Geometry check sheet. Reference: the model listing, model coordinates, mm. Face numbers are marked on the shaded views. A direction names the side the tool comes from. Round coordinates to 2 decimals unless told otherwise and drop trailing zeros. Loops run counter-clockwise (first coordinate to the right, second up) from the corner with the lowest first, then second, coordinate; pieces in that order, holes last. Notation, with made-up numbers: (50.25, -23.75) - (84.25, -23.75) arc R16 cw to (84.25, -18.75) - close; hole circle Ø1 at (32.25, -33.75). An arc over 180 degrees is marked (long way). Write item = value, one per line.
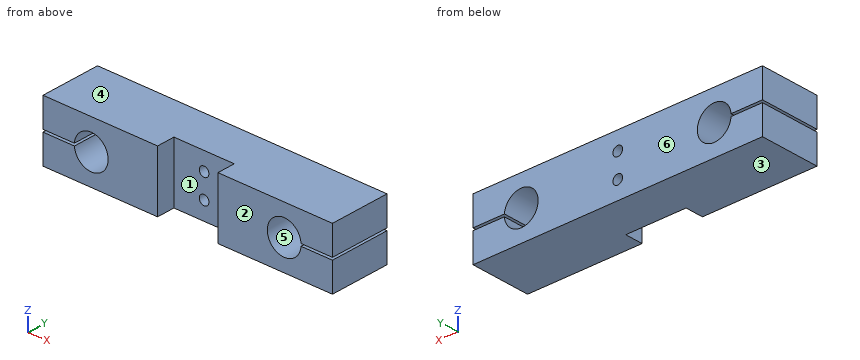
```python
from build123d import *

# Parameters (mm, degrees)
EXTRUDE_1_DEPTH     = 50
SKETCH_3_W          = 50
SKETCH_3_H          = 50
CUT_EXTRUDE_1_DEPTH = 15
SKETCH_4_R          = 4
CUT_EXTRUDE_2_DEPTH = 50


with BuildPart() as part:
    # Эскиз1 → Бобышка-Вытянуть1 (new body)
    with BuildSketch(Plane(origin=(0, 0, 0), x_dir=(1, 0, 0), z_dir=(0, 1, 0))):
        with BuildLine():
            Line((0, 0), (240, 0))
            Line((240, 0), (240, 24))
            Line((240, 24), (213.964240044, 24))
            ThreePointArc((213.964240044, 24), (186, 25), (213.964240044, 26))
            Line((213.964240044, 26), (240, 26))
            Line((240, 26), (240, 50))
            Line((240, 50), (0, 50))
            Line((0, 50), (0, 26))
            Line((0, 26), (26.035759956, 26))
            ThreePointArc((26.035759956, 26), (54, 25), (26.035759956, 24))
            Line((26.035759956, 24), (0, 24))
            Line((0, 24), (0, 0))
        make_face()
    extrude(amount=EXTRUDE_1_DEPTH)

    # Эскиз3 → Вырез-Вытянуть1 (cut)
    with BuildSketch(Plane.XZ):
        with Locations((120, -25)):
            Rectangle(SKETCH_3_W, SKETCH_3_H)
    extrude(amount=-CUT_EXTRUDE_1_DEPTH, mode=Mode.SUBTRACT)

    # Эскиз4 → Вырез-Вытянуть2 (cut)
    with BuildSketch(Plane(origin=(0, 50, 0), x_dir=(1, 0, 0), z_dir=(0, 1, 0))):
        with Locations(Location((120, 35, 0), (0, 0, 270))):
            Circle(SKETCH_4_R)
        with Locations(Location((120, 15, 0), (0, 0, 270))):
            Circle(SKETCH_4_R)
    extrude(amount=-CUT_EXTRUDE_2_DEPTH, mode=Mode.SUBTRACT)


solid = part.part
```
(1) Mould release check, pull along Z, two halves, no side actions. Record for the marked faces 3, 4, 5 and 6: pulls with the +Z half, pulls with the -Z half, needs draft (parallel to the pull), parting line crosses it, or undercut.
Answers follow:
face_3 = pulls with the -Z half
face_4 = pulls with the +Z half
face_5 = undercut
face_6 = needs draft
(2) Section check B-B (y = 21). Enter the section's corners in (x, z).
Answers follow:
outline = (0, -50) - (240, -50) - (240, -26) - (213.96, -26) arc R14 cw (long way) to (213.96, -24) - (240, -24) - (240, 0) - (0, 0) - (0, -24) - (26.04, -24) arc R14 cw (long way) to (26.04, -26) - (0, -26) - close; hole circle Ø8 at (120, -35); hole circle Ø8 at (120, -15)
(3) Set-up check for the marked faces 1 and 2: record each of +Z, -Z, +X, -X, +Y, -Y from which the full face is reachable in a straight line by a thin tool's end or side.
Answers follow:
face_1 = +Z, -Z, -Y
face_2 = +Z, -Z, +X, -X, -Y
(4) Section check C-C (x = 200). Enter the section's corners in (y, z), then the cut area to 3 significant figures.
Answers follow:
outline = (0, -50) - (50, -50) - (50, -39) - (0, -39) - close; (0, -11) - (50, -11) - (50, 0) - (0, 0) - close
area = 1,100 mm²
(5) Section check A-A (x = 120). Enter the section's corners in (y, z), then the cut area to 3 significant figures.
Answers follow:
outline = (15, -50) - (50, -50) - (50, -39) - (15, -39) - close; (15, -31) - (50, -31) - (50, -19) - (15, -19) - close; (15, -11) - (50, -11) - (50, 0) - (15, 0) - close
area = 1,190 mm²
(6) Section check D-D (z = -5). Enter the section's corners in (x, y), then the cut area to 4 significant figures.
Answers follow:
outline = (0, 0) - (95, 0) - (95, 15) - (145, 15) - (145, 0) - (240, 0) - (240, 50) - (0, 50) - close
area = 11,250 mm²
(7) Scan lines: L1, parallel to Z at x = 200, y = 39.5; L2, parallel to X at y = 28, z = -15; L3, parallel to X at y = 45, z = -22. Record each from-to range of solid material in increasing order. Write a range as [from, to].
Answers follow:
L1 = [-50, -39], [-11, 0]
L2 = [0, 30.2], [49.8, 116], [124, 190.2], [209.8, 240]
L3 = [0, 26.33], [53.67, 186.33], [213.67, 240]
(8) Gauge pin test, flat ends, axial feed: pin 1 (9 mm diameter, centred on x = 120, z = -15, fed in from -Y); pin 2 (1.5 mm diameter, centred on y = 10, z = -44, fed in from -X). Record the tip position at first contact, or that the pin passes through.
Answers follow:
pin_1 = 15
pin_2 = 0
